The listing builds one solid part. Answer for the finished solid, in the listing's coordinates (mm). A direction names the side the tool comes from. Give positions to 0.01 mm unless a question says otherwise; leave off trailing zeros. Loops run counter-clockwise (first coordinate to the right, second up) from the corner with the lowest first, then second, coordinate; pieces in that order, holes last. Notation, with made-up numbers: M 5,18 L 62,18 A27 cw 62,40 Z; hole C 6,69 d8. An arc over 180 degrees is marked long. One line per item, written item: value. Start each with the question number.
Q1. A cutting plane is placed at A-A, the plane x = 9. Determine the outline of the cut face in (y, z), and give its area (3 significant figures).
Q2. The mould has two halves that part along Y. Classify faces 1 (the flat face through (7, 0, 27)), 2 (the cylindrical face through (7.94, -228.89, 32.07)), 3 (the flat face through (6, -154, 19.201)): +Y half, -Y half, draft (parallel to the pull), parting line (faces both ways), or undercut.
Q3. A flat-ended cylindrical pin translates along its axis: pin 1 (6.5 mm diameter, centred on y = -228.19, z = 26.78, fed in from -X). Find the tip coordinate at first contact, or state that the pin passes through.
Q4. Consider L1, parallel to Y at x = 20, z = 26.5; L2, parallel to Y at x = 7.5, z = 20.5; L3, parallel to X at y = -208, z = 32. Determine where each line is inside the solid, lowest interval first.
Q5. For faces 4 (the flat face through (6, -313, 27)), 5 (the flat face through (-12.644, -158, 33)), determine the directions among +Z, -Z, +X, -X, +Y, -Y from which every point of the face is accessible in a straight line to the end or side of a thin tool.
Q6. A cutting plane is placed at C-C, the plane y = -269. Determine the outline of the cut face in (x, z).
Q7. A cutting plane is placed at B-B, the plane x = -7.5. Determine the outline of the cut face in (y, z), and give its area (3 significant figures).
from build123d import *

# Parameters (mm, degrees)
F0_W     = 63.378432
F0_H     = 16.102
F1_DEPTH = 313
F2_R     = 5.335787
F3_DEPTH = 63.379432
F5_R     = 4.717458
F6_DEPTH = 25
F8_DEPTH = 25
F9_DEPTH = 25


with BuildPart() as f1:
    # F0 (on Front) → F1 (new body)
    with BuildSketch(Plane.XZ):
        with Locations((-3.735943, 27.252212)):
            Rectangle(F0_W, F0_H)
    extrude(amount=F1_DEPTH)

    # F2 (on face) → F3 (cut, through all)
    with BuildSketch(Plane.YZ.offset(27.953273)):
        with Locations((-18.191617, 26.778789)):
            Circle(F2_R)
        with Locations((-88.191617, 26.778789)):
            Circle(F2_R)
        with Locations((-158.191617, 26.778789)):
            Circle(F2_R)
        with Locations((-228.191617, 26.778789)):
            Circle(F2_R)
        with Locations((-298.191617, 26.778789)):
            Circle(F2_R)
    extrude(amount=-F3_DEPTH, mode=Mode.SUBTRACT)

    # F5 (on face) → F6 (cut)
    with BuildSketch(Plane(origin=(0, 0, 19.201212), x_dir=(1, 0, 0), z_dir=(0, 0, -1))):
        with Locations((8.254815, 6.340917)):
            Circle(F5_R)
    extrude(amount=-F6_DEPTH, mode=Mode.SUBTRACT)

    # F7 (on face) → F8 (cut)
    with BuildSketch(Plane.XY.offset(35.303212)):
        Polygon((-34.219209, -324.690997), (-12.643897, -311.831832), (-12.643897, 0), (-35.135265, 11.57862), (-57.62665, 0), (-81.669144, -321.138591), align=None)
    extrude(amount=-F8_DEPTH, mode=Mode.SUBTRACT)

    # F5 (on face) → F9 (cut)
    with BuildSketch(Plane(origin=(0, 0, 19.201212), x_dir=(1, 0, 0), z_dir=(0, 0, -1))):
        with Locations((8.254815, 6.340917)):
            Circle(F5_R)
    extrude(amount=-F9_DEPTH, mode=Mode.SUBTRACT)


solid = f1.part
Answer block:
1. outline: M -313,19.2 L -11,19.2 L -11,35.3 L -313,35.3 Z; M -1.68,19.2 L 0,19.2 L 0,35.3 L -1.68,35.3 Z; hole C -298.19,26.78 d10.67; hole C -228.19,26.78 d10.67; hole C -158.19,26.78 d10.67; hole C -88.19,26.78 d10.67; hole C -18.19,26.78 d10.67
1. area: 4,440 mm^2
2. face 1: +Y half
2. face 2: undercut
2. face 3: draft
3. pin 1: through
4. L1: -313 to -303.52, -292.86 to -233.52, -222.86 to -163.52, -152.86 to -93.52, -82.86 to -23.52, -12.86 to 0
4. L2: -313 to -11, -1.68 to 0
4. L3: -12.64 to 27.95
5. face 4: +Z, -Z, +X, -X, -Y
5. face 5: +Z, -Z, -X, +Y
6. outline: M -12.64,19.2 L 27.95,19.2 L 27.95,35.3 L -12.64,35.3 Z
7. outline: M -313,19.2 L 0,19.2 L 0,35.3 L -313,35.3 Z; hole C -298.19,26.78 d10.67; hole C -228.19,26.78 d10.67; hole C -158.19,26.78 d10.67; hole C -88.19,26.78 d10.67; hole C -18.19,26.78 d10.67
7. area: 4,590 mm^2
